from build123d import *

# Parameters (mm, degrees)
SKETCH1_R                       = 44.45
SKETCH1_R_2                     = 39.6875
BOSS_EXTRUDE1_DEPTH             = 209.55
SKETCH2_W                       = 7.89975339
SKETCH2_H                       = 28.462346772
CUT_EXTRUDE1_DEPTH              = 38.1
F_10_32_TAPPED_HOLE1_AT_2_COUNT = 2
F_10_32_TAPPED_HOLE1_AT_2_PITCH = 12.7
F_6_32_TAPPED_HOLE1_D           = 2.7051
F_6_32_TAPPED_HOLE1_DEPTH       = 14.986
F_6_32_TAPPED_HOLE1_TIP         = 0.81269403
F_6_32_TAPPED_HOLE2_REACH       = 408.053
F_6_32_TAPPED_HOLE2_BORE_R      = 1.35255
CIRPATTERN1_COUNT               = 3


with BuildPart() as part:
    # Sketch1 → Boss-Extrude1 (new, symmetric)
    with BuildSketch(Plane.XY):
        Circle(SKETCH1_R)
        Circle(SKETCH1_R_2, mode=Mode.SUBTRACT)
    extrude(amount=BOSS_EXTRUDE1_DEPTH, both=True)

    # Sketch2 → Cut-Extrude1 (cut)
    with BuildSketch(Plane.XY.offset(209.55)):
        with Locations((47.129876695, -0.406604954)):
            Rectangle(SKETCH2_W, SKETCH2_H)
    cut_extrude1 = extrude(amount=-CUT_EXTRUDE1_DEPTH, mode=Mode.SUBTRACT)

    # Sketch3 → 10-32 Tapped Hole1 (revolve, cut)
    with BuildSketch(Plane(origin=(43.18, 0, 200.025), x_dir=(0, 0, -1), z_dir=(0, 1, 0))):
        Polygon((0, 0), (0, 14.929317848), (2.0193, 13.716), (2.0193, 0), align=None)
    f_10_32_tapped_hole1 = revolve(axis=Axis((49.53, 0, 200.025), (-1, 0, 0)), mode=Mode.SUBTRACT)

    # 10-32 Tapped Hole1 at 2: 10-32 Tapped Hole1 ×2
    with Locations(*[(0, 0, -i * F_10_32_TAPPED_HOLE1_AT_2_PITCH) for i in range(1, F_10_32_TAPPED_HOLE1_AT_2_COUNT)]):
        add(f_10_32_tapped_hole1, mode=Mode.SUBTRACT)

    # 6-32 Tapped Hole1
    with Locations(Plane(origin=(0, 0, -209.55), x_dir=(-1, 0, 0), z_dir=(0, 0, -1))):
        with Locations((0, 42.06875), (-42.06875, 0), (42.06875, 0), (0, -42.06875)):
            Hole(F_6_32_TAPPED_HOLE1_D / 2, depth=F_6_32_TAPPED_HOLE1_DEPTH)
            with Locations((0, 0, -(F_6_32_TAPPED_HOLE1_DEPTH + F_6_32_TAPPED_HOLE1_TIP / 2))):  # 118° drill point
                Cone(0, F_6_32_TAPPED_HOLE1_D / 2, F_6_32_TAPPED_HOLE1_TIP, mode=Mode.SUBTRACT)

    # Mirror1: Cut-Extrude1, 10-32 Tapped Hole1 across plane
    add(cut_extrude1.mirror(Plane(origin=(0, 0, 0), x_dir=(0, 0, 1), z_dir=(1, 0, 0))), mode=Mode.SUBTRACT)
    add(f_10_32_tapped_hole1.mirror(Plane(origin=(0, 0, 0), x_dir=(0, 0, 1), z_dir=(1, 0, 0))), mode=Mode.SUBTRACT)

    # Mirror1 copy 1 sketch → Mirror1 copy 1 (revolve, cut)
    with BuildSketch(Plane(origin=(-43.18, 0, 187.325), x_dir=(0, 0, -1), z_dir=(0, 1, 0))):
        Polygon((0, 0), (0, -14.929317848), (2.0193, -13.716), (2.0193, 0), align=None)
    revolve(axis=Axis((-49.53, 0, 187.325), (-1, 0, 0)), mode=Mode.SUBTRACT)

    # 6-32 Tapped Hole2 bore (on position points) → 6-32 Tapped Hole2 (cut, up to next)
    with BuildSketch(Plane(origin=(0, 44.45, -184.15), x_dir=(1, 0, 0), z_dir=(0, 1, 0)), mode=Mode.PRIVATE) as f_6_32_tapped_hole2_sk1:
        Circle(F_6_32_TAPPED_HOLE2_BORE_R)
    f_6_32_tapped_hole2_tool1 = extrude(f_6_32_tapped_hole2_sk1.sketch, amount=-F_6_32_TAPPED_HOLE2_REACH, mode=Mode.PRIVATE) & part.part
    # 6-32 Tapped Hole2 bore (on position points) → 6-32 Tapped Hole2 (cut, up to next)
    with BuildSketch(Plane(origin=(0, 44.45, -184.15), x_dir=(1, 0, 0), z_dir=(0, 1, 0)), mode=Mode.PRIVATE) as f_6_32_tapped_hole2_sk2:
        with Locations((0, -292.1)):
            Circle(F_6_32_TAPPED_HOLE2_BORE_R)
    f_6_32_tapped_hole2_tool2 = extrude(f_6_32_tapped_hole2_sk2.sketch, amount=-F_6_32_TAPPED_HOLE2_REACH, mode=Mode.PRIVATE) & part.part
    f_6_32_tapped_hole2_1 = f_6_32_tapped_hole2_tool1.solids().sort_by_distance((0, 44.45, -184.15))[0]
    add(f_6_32_tapped_hole2_1, mode=Mode.SUBTRACT)
    f_6_32_tapped_hole2_2 = f_6_32_tapped_hole2_tool2.solids().sort_by_distance((0, 44.45, 107.95))[0]
    add(f_6_32_tapped_hole2_2, mode=Mode.SUBTRACT)
    f_6_32_tapped_hole2 = f_6_32_tapped_hole2_1 + f_6_32_tapped_hole2_2  # 6-32 Tapped Hole2 as one shape, for the pattern or mirror that repeats it

    # CirPattern1: 6-32 Tapped Hole2 ×3 about axis
    cirpattern1_axis = Axis((0, 0, -209.55), (0, 0, 1))
    for i in range(1, CIRPATTERN1_COUNT):
        add(f_6_32_tapped_hole2.rotate(cirpattern1_axis, i * 360 / CIRPATTERN1_COUNT), mode=Mode.SUBTRACT)


solid = part.part
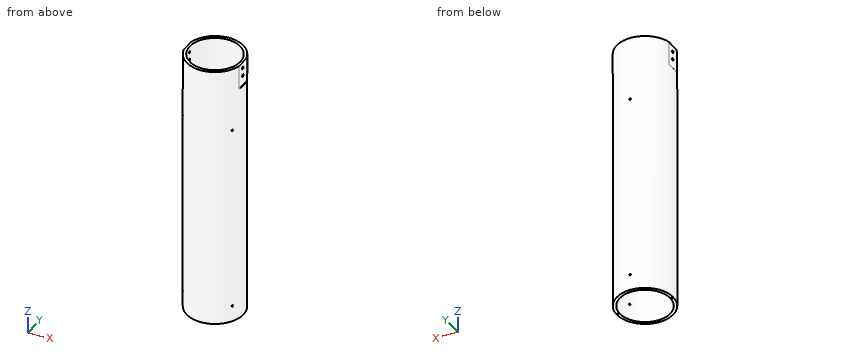
The listing builds one solid part. Answer for the finished solid, in the listing's coordinates (mm). Coordinates: 2 decimals unless noted, no trailing zeros. Write each loop counter-clockwise with the first axis right and the second up, starting at its lowest first coordinate (ties: lowest second). Pieces come first, ordered by that corner, then holes. Notation, with made-up numbers: M 45,10.5 L 54,10.5 A22 ccw 54,27.5 Z; hole C 62,-24.75 d4. An arc over 180 degrees is marked long. Put each result on its own line as item: value. Start each with the question number.
1. A cutting plane is placed at A-A on x = -27. Write down the section's boundary in (y, z), then the cut area to 3 significant figures.
2. A cutting plane is placed at B-B on y = 25. Write down the section's boundary in (x, z), then the cut area to 3 significant figures.
3. Flat-ended cylindrical pins translate along their axes: P1, Ø12, axis at y = 20, z = -53.5, coming from the +X side; P2, Ø5.5, axis at y = 0, z = 187.325, coming from the +X side; P3, Ø6, axis at y = 14, z = 122, coming from the +X side; P4, Ø10, axis at x = -29, y = 16, coming from the +Z side. Find the tip coordinate at first contact, or state that the pin passes through.
4. Consider line 1 (X direction, y = -2, z = -68); line 2 (X direction, y = 22, z = -67.5). Determine where each line is inside the solid, lowest interval first. Write a range as from..to.
Resolved:
1. outline: M -35.31,-209.55 L -29.09,-209.55 L -29.09,209.55 L -35.31,209.55 Z; M 29.09,-209.55 L 35.31,-209.55 L 35.31,209.55 L 29.09,209.55 Z
1. area: 5,220 mm2
2. outline: M -36.75,-209.55 L -30.82,-209.55 L -30.82,209.55 L -36.75,209.55 Z; M 30.82,-209.55 L 36.75,-209.55 L 36.75,209.55 L 30.82,209.55 Z
2. area: 4,970 mm2
3. P1: stops at x = 42.19
3. P2: stops at x = 43.18
3. P3: stops at x = 43.07
3. P4: passes through
4. line 1: x = -44.4..-39.64, 39.64..44.4
4. line 2: x = -38.62..-33.03, 33.03..38.62
